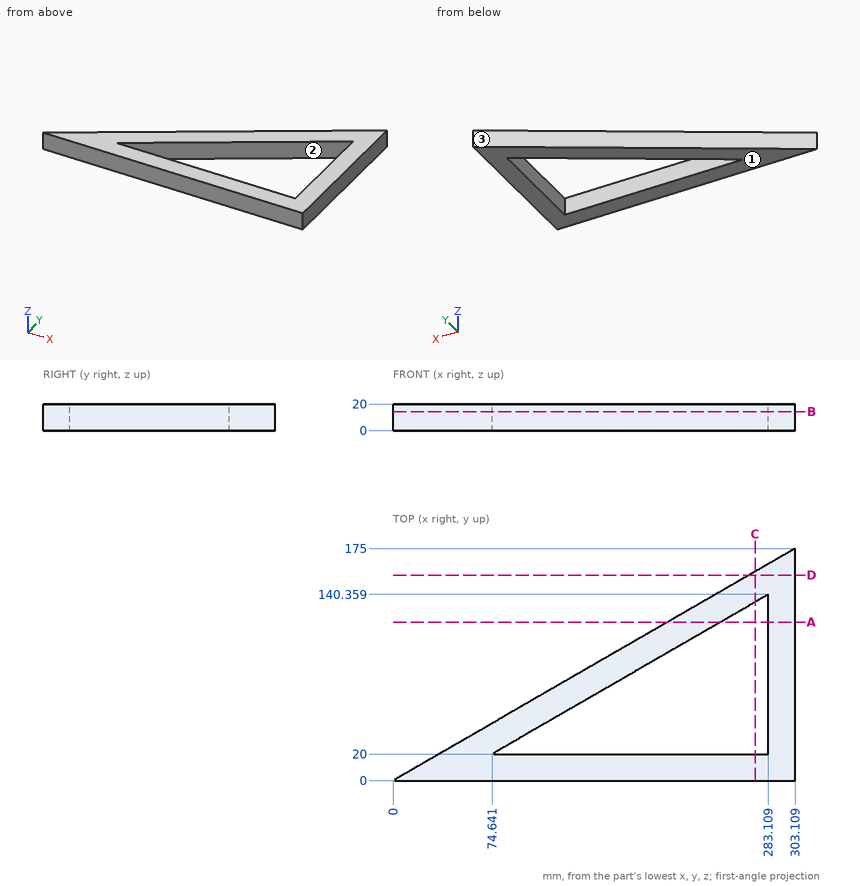
Study the drawing (mm; zero at the part's minimum x, y, z) and answer. Give positions to 0.01 mm unless a question says otherwise; leave off trailing zeros. Order: outer loops, then holes, each group sorted by start corner. A loop starts at its lowest first (then second) coordinate and runs counter-clockwise, first axis right, second up.
1. The mould has two halves that part along X. Classify the marked faces 1, 2 and 3: released by +X, released by -X, zero draft, split by the parting line, or undercut.
Result sheet:
face 1: zero draft
face 2: undercut
face 3: released by -X
2. Section C-C, the plane x = 273 is taken. Determine the outline of the cut face in (y, z).
Result sheet:
outline: (0, 0) - (20, 0) - (20, 20) - (0, 20) - close; (134.52, 0) - (157.62, 0) - (157.62, 20) - (134.52, 20) - close
3. Each of these flat-tipped pins is pushed along its axis until it touches: P1, Ø5, axis at x = 60, z = 12, coming from the +Y side; P2, Ø6, axis at x = 237.5, z = 12, coming from the +Y side; P3, Ø6, axis at y = 137, z = 15, coming from the -X side (1 decimal). Where does it stop, or does it pass through?
Result sheet:
P1: stops at y = 36.08
P2: stops at y = 138.85
P3: stops at x = 232.1
4. Section A-A, the plane y = 119.5 is taken. Determine the outline of the cut face in (x, z), and give its area (3 significant figures).
Result sheet:
outline: (206.98, 0) - (246.98, 0) - (246.98, 20) - (206.98, 20) - close; (283.11, 0) - (303.11, 0) - (303.11, 20) - (283.11, 20) - close
area: 1,200 mm2
5. Straight lines are drawn through the part: L1, parallel to X at y = 95, z = 5.25 (1 decimal); L2, parallel to X at y = 114, z = 1; L3, parallel to Y at x = 223.5, z = 9.5. For each, find the intervals that lie inside material, in ascending order.
Result sheet:
L1: x = 164.5 to 204.5, 283.1 to 303.1
L2: x = 197.45 to 237.45, 283.11 to 303.11
L3: y = 0 to 20, 105.94 to 129.04
6. Section B-B, the plane z = 14.25 is taken. Determine the outline of the cut face in (x, y).
Result sheet:
outline: (0, 0) - (303.11, 0) - (303.11, 175) - close; hole (74.64, 20) - (283.11, 20) - (283.11, 140.36) - close
7. Section D-D, the plane y = 155 is taken. Determine the outline of the cut face in (x, z).
Result sheet:
outline: (268.47, 0) - (303.11, 0) - (303.11, 20) - (268.47, 20) - close
